```python
from build123d import *

# Parameters (mm, degrees)
SKETCH_R         = 2.05
EXTRUDE001_DEPTH = 5
CHAMFER_SIZE     = 2
SKETCH001_R      = 3
POCKET_DEPTH     = 2


with BuildPart() as part:
    # Sketch → Extrude001 (new body)
    with BuildSketch(Plane.XY):
        Polygon((0, 0), (0, 40), (20, 40), (40, 20), (40, 0), align=None)
        with Locations((10, 10)):
            Circle(SKETCH_R, mode=Mode.SUBTRACT)
        with Locations((10, 30)):
            Circle(SKETCH_R, mode=Mode.SUBTRACT)
        with Locations((30, 10)):
            Circle(SKETCH_R, mode=Mode.SUBTRACT)
    extrude(amount=EXTRUDE001_DEPTH)

    # Chamfer
    chamfer_edges = [part.edges().sort_by_distance(p)[0] for p in [
        (0, 20, 5),
        (10, 40, 5),
        (30, 30, 5),
        (40, 10, 5),
        (20, 0, 5),
    ]]
    chamfer(chamfer_edges, length=CHAMFER_SIZE)

    # Sketch001 → Pocket (cut)
    with BuildSketch(Plane.XY.offset(5)):
        with Locations((10, 30)):
            Circle(SKETCH001_R)
        with Locations((10, 10)):
            Circle(SKETCH001_R)
        with Locations((30, 10)):
            Circle(SKETCH001_R)
    extrude(amount=-POCKET_DEPTH, mode=Mode.SUBTRACT)


solid = part.part
```
Here's how the part is built. I have some questions about the finished solid (model axes, mm). A direction names the side the tool comes from. Give positions to 0.01 mm unless a question says otherwise; leave off trailing zeros. Loops run counter-clockwise (first coordinate to the right, second up) from the corner with the lowest first, then second, coordinate; pieces in that order, holes last. Notation, with made-up numbers: M -22,63.25 L 0,63.25 A17 ccw 0,95.25 Z; hole C 42.25,27.25 d3. An arc over 180 degrees is marked long. Return JSON: item names as keys, results as strings.
Item 1: Thinking about a two-plate mould opening in Y: for faces 1 (the flat face through (10, 39, 4)), 2 (the flat face through (20, 0, 1)), 3 (the flat face through (40, 10, 1)), 4 (the cylindrical face through (28.373, 8.753, 1.479)), which applies, released by +Y, released by -Y, zero draft, split by the parting line, or undercut?
A:
{"face 1": "released by +Y", "face 2": "released by -Y", "face 3": "zero draft", "face 4": "undercut"}
Item 2: Imagine slicing it at C-C on z = 1.55. List the corners of the cut face in (x, y) for me, then the cut area to 3 significant figures.
A:
{"outline": "M 0,0 L 40,0 L 40,20 L 20,40 L 0,40 Z; hole C 10,10 d4.1; hole C 10,30 d4.1; hole C 30,10 d4.1", "area": "1,360 mm^2"}
Item 3: On a 3-axis mill with a long thin cutter (end or side, diameter ignored), from which of +Z, -Z, +X, -X, +Y, -Y can I reach the whole of each face in a straight line? I mean faces 5 (the flat face through (1, 20, 4)), 6 (the flat face through (32, 9, 3)). Say none if no direction works.
A:
{"face 5": "+Z, -X, +Y, -Y", "face 6": "+Z"}
Item 4: I'm going to push flat-ended pins straight in: pin 1 Ø2 at (y, z) = (24.5, 3.5) entering from +X; pin 2 Ø1.5 at (x, z) = (26, 3.5) entering from +Y; pin 3 Ø5 at (x, y) = (10, 10) entering from +Z; pin 4 Ø3.5 at (x, y) = (30, 10) entering from -Z. Where does each tip first touch, or does it pass through?
A:
{"pin 1": "stops at x = 36.37", "pin 2": "stops at y = 34.56", "pin 3": "stops at z = 3", "pin 4": "passes through"}
Item 5: Imagine slicing it at A-A on x = 10. List the corners of the cut face in (y, z) for me.
A:
{"outline": "M 0,0 L 7.95,0 L 7.95,3 L 7,3 L 7,5 L 2,5 L 0,3 Z; M 12.05,0 L 27.95,0 L 27.95,3 L 27,3 L 27,5 L 13,5 L 13,3 L 12.05,3 Z; M 32.05,0 L 40,0 L 40,3 L 38,5 L 33,5 L 33,3 L 32.05,3 Z"}
Item 6: Imagine slicing it at D-D on x = 31.5. List the corners of the cut face in (y, z) for me.
A:
{"outline": "M 0,0 L 8.6,0 L 8.6,3 L 7.4,3 L 7.4,5 L 2,5 L 0,3 Z; M 11.4,0 L 28.5,0 L 28.5,3 L 25.67,5 L 12.6,5 L 12.6,3 L 11.4,3 Z"}
Item 7: Please list where these lines run through material, in increasing order: line 1 (Y direction, x = 10, z = 2.15); line 2 (Y direction, x = 10, z = 3.7).
A:
{"line 1": "y = 0 to 7.95, 12.05 to 27.95, 32.05 to 40", "line 2": "y = 0.7 to 7, 13 to 27, 33 to 39.3"}
